Check sheet for the modelled part. Datum: model origin and axes. Units: mm. A direction names the side the tool comes from. Give positions to 0.01 mm unless a question says otherwise; leave off trailing zeros. Write each loop counter-clockwise with the first axis right and the second up, starting at its lowest first coordinate (ties: lowest second). Pieces come first, ordered by that corner, then holes. Notation, with made-up numbers: (80.5, 81) -> (131.5, 81) arc R23 cw to (131.5, 100) -> close; hole circle Ø6 at (40.25, 36). An arc over 180 degrees is marked (long way). Answer as a JSON object with one key per item and string values.
from build123d import *

# Parameters (mm, degrees)
SKETCH1_R            = 28.575
CONE_EXTRUDE_DEPTH   = 25.4
CONE_EXTRUDE_TAPER   = 25
MOTOR_AXLE_CUT_DEPTH = 15.25
CHAMFER1_SIZE        = 2
CHAMFER1_SIZE_2      = 4.134883836
CHAMFER2_SIZE        = 2
BOLT_HOLE_CUT_DEPTH  = 5.08
FILLET1_R            = 0.635


with BuildPart() as part:
    # Sketch1 → Cone Extrude (new body)
    with BuildSketch(Plane.XY):
        Circle(SKETCH1_R)
    extrude(amount=CONE_EXTRUDE_DEPTH, taper=CONE_EXTRUDE_TAPER)

    # Sketch2 → Motor Axle Cut (cut)
    with BuildSketch(Plane(origin=(0, 0, 0), x_dir=(-1, 0, 0), z_dir=(0, 0, -1))):
        with BuildLine():
            Line((-2.059884706, 2.35), (2.059884706, 2.35))
            ThreePointArc((2.059884706, 2.35), (0, -3.125), (-2.059884706, 2.35))
        make_face()
    extrude(amount=-MOTOR_AXLE_CUT_DEPTH, mode=Mode.SUBTRACT)

    # Chamfer1
    # the kernel refuses this chamfer: 4.134883836, 2 mm, written as the material it takes off along each edge
    with BuildSketch(Plane(origin=(0, 0, 25.4), x_dir=(1, 0, 0), z_dir=(0, 1, 0))) as chamfer1_piece_1:
        Polygon((16.730785483 + CHAMFER1_SIZE * 0.422618261741, CHAMFER1_SIZE * 0.906307787037), (16.730785483 - CHAMFER1_SIZE_2, 0), (16.730785483, 0), align=None)
    revolve(axis=Axis((0, 0, 25.4), (0, 0, -1)), mode=Mode.SUBTRACT)

    # Chamfer2
    chamfer2_edges = [part.edges().sort_by_distance(p)[0] for p in [
        (0, -3.125, 0),
        (0, 2.35, 0),
    ]]
    chamfer(chamfer2_edges, length=CHAMFER2_SIZE)

    # Sketch3 → Bolt Hole Cut (cut)
    with BuildSketch(Plane.XY.offset(25.4)):
        Polygon((6.741570116, 5.654240212), (-1.525930605, 8.665491088), (-8.267500721, 3.011250876), (-6.741570116, -5.654240212), (1.525930605, -8.665491088), (8.267500721, -3.011250876), align=None)
    extrude(amount=-BOLT_HOLE_CUT_DEPTH, mode=Mode.SUBTRACT)

    # Fillet1
    fillet1_edges = [part.edges().sort_by_distance(p)[0] for p in [
        (-28.575, 0, 0),
    ]]
    fillet(fillet1_edges, radius=FILLET1_R)


solid = part.part
1. Mould release check, pull along X, two halves, no side actions. Record for faces 4 (the face through (18.375, 5.787, 19.966)), 5 (the face through (-0.2, -8.2, 25.4)), 6 (the face through (7.515, 1.261, 22.896)): released by +X, released by -X, zero draft, split by the parting line, or undercut.
Determined:
{"face 4": "split by the parting line", "face 5": "zero draft", "face 6": "undercut"}
2. Sectioned sample at C-C, the plane z = 13.25. Enter the section's corners in (x, y) (3 decimals).
Determined:
{"outline": "circle Ø44.793 at (0, 0); hole (-2.06, 2.35) arc R3.125 ccw (long way) to (2.06, 2.35) -> close"}
3. Scan lines: L1, parallel to Z at x = -4.5, y = -3.5; L2, parallel to X at y = 5, z = 22.5; L3, parallel to X at y = 0, z = 7 (3 decimals). Record each from-to range of solid material in increasing order. Write a range as [from, to].
Determined:
{"L1": "[0, 20.32]", "L2": "[-17.38, -5.9], [6.86, 17.38]", "L3": "[-25.311, -3.125], [3.125, 25.311]"}
4. Sectioned sample at A-A, the plane x = 0. Enter the section's corners in (y, z) (3 decimals), plus the area to 3 significant figures.
Determined:
{"outline": "(-28.154, 0.903) arc R0.635 ccw to (-27.578, 0) -> (-5.125, 0) -> (-3.125, 2) -> (-3.125, 15.25) -> (2.35, 15.25) -> (2.35, 2) -> (4.35, 0) -> (27.578, 0) arc R0.635 ccw to (28.154, 0.903) -> (17.576, 23.587) -> (12.596, 25.4) -> (8.11, 25.4) -> (8.11, 20.32) -> (-8.11, 20.32) -> (-8.11, 25.4) -> (-12.596, 25.4) -> (-17.576, 23.587) -> close", "area": "973 mm^2"}
5. Sectioned sample at B-B, the plane y = 0. Enter the section's corners in (x, z) (3 decimals).
Determined:
{"outline": "(-28.154, 0.903) arc R0.635 ccw to (-27.578, 0) -> (-5.125, 0) -> (-3.125, 2) -> (-3.125, 15.25) -> (3.125, 15.25) -> (3.125, 2) -> (5.125, 0) -> (27.578, 0) arc R0.635 ccw to (28.154, 0.903) -> (17.576, 23.587) -> (12.596, 25.4) -> (7.737, 25.4) -> (7.737, 20.32) -> (-7.737, 20.32) -> (-7.737, 25.4) -> (-12.596, 25.4) -> (-17.576, 23.587) -> close"}
6. Sectioned sample at D-D, the plane z = 9.25. Enter the section's corners in (x, y) (3 decimals), plus the area to 3 significant figures.
Determined:
{"outline": "circle Ø48.523 at (0, 0); hole (-2.06, 2.35) arc R3.125 ccw (long way) to (2.06, 2.35) -> close", "area": "1,820 mm^2"}
7. Go/stop test with flat-tipped pins: P1, Ø5.5, axis at x = 0, y = 0, coming from the +Z side; P2, Ø3, axis at y = -3, z = 12, coming from the +X side; P3, Ø10, axis at x = 8.5, y = -22.5, coming from the +Z side. Record where each tip stops, or that it passes through.
Determined:
{"P1": "z = 20.32", "P2": "x = 23.51", "P3": "z = 20.42"}
8. Access from +Z, -Z, +X, -X, +Y, -Y to the whole of each face (thin tool, end or side, straight path). Record for faces 1 (the face through (-0.106, -3.123, 8.532)), 2 (the face through (6, 0, 0)), 3 (the face through (-2.666, -7.139, 22.896)).
Determined:
{"face 1": "-Z", "face 2": "-Z, +X, -X, +Y, -Y", "face 3": "+Z"}
